Here's how the part is built. I have some questions about the finished solid (model axes, mm). A direction names the side the tool comes from. Round coordinates to 2 decimals unless told otherwise and drop trailing zeros. Write each loop counter-clockwise with the first axis right and the second up, starting at its lowest first coordinate (ties: lowest second). Pieces come first, ordered by that corner, then holes. Notation, with made-up numbers: M 33.5,38 L 62.5,38 A16 cw 62.5,64 Z; hole C -29.5,20 d1. An arc over 180 degrees is marked long. Use one line per item in the form item = value. Start each with the question number.
Q1. We'd pull the mould along X, two halves only. Please class faces 5 (the face through (-10, 82, -13)), 6 (the face through (60, 1, 0)), 7 (the face through (-1, 33, 22)): +X half, -X half, draft (parallel to the pull), parting line (faces both ways), or undercut.
Q2. For faces 1 (the face through (-42, 25, -5)), 2 (the face through (-45, 28, -6)), 3 (the face through (53, 3, 0)), 4 (the face through (-40, 66, -11)), which set-ups out of +Z, -Z, +X, -X, +Y, -Y let a thin tool reach every point of the face, with its end or its side?
Q3. I want a section at B-B on z = -17.5. List the corners of the cut face in (x, y) for me, and give its area (3 significant figures).
Q4. I want a section at C-C on y = 23. List the corners of the cut face in (x, z) for me.
Q5. I need wall thicknesses on line 1 along Z through (x, y) = (-52.5, 2.3); line 2 along X through (y, z) = (1.85, -17.5); line 3 along Y through (x, z) = (0, -24). Which ranges of each line are inside material? Lowest first, please. Write a range as from..to.
Q6. I'm going to push flat-ended pins straight in: pin 1 Ø8 at (y, z) = (14.5, -16) entering from +X; pin 2 Ø4 at (x, z) = (-42, 1.5) entering from +Y; pin 3 Ø10 at (y, z) = (37, -13.5) entering from -X. Where does each tip first touch, or does it pass through?
Q7. I want a section at D-D on z = 8. List the corners of the cut face in (x, y) for me (3 decimals), and give its area (3 significant figures).
Q8. I want a section at A-A on x = 52.5. List the corners of the cut face in (y, z) for me.
Autodesk Inventor part; units mm, degrees
ref_plane "YZ Plane" through (0, 0, 0) normal (1, 0, 0) x (0, 1, 0)
ref_plane "XZ Plane" through (0, 0, 0) normal (0, 1, 0) x (-1, 0, 0)
ref_plane "XY Plane" through (0, 0, 0) normal (0, 0, 1) x (1, 0, 0)
sketch "Skizze1" plane through (0, 0, 0) normal (0, 1, 0) x (-1, 0, 0)
  line L0 (60, 25) -> (-60, 25)
  line L1 (-60, 25) -> (-60, -25)
  line L2 (-60, -25) -> (60, -25)
  line L3 (60, -25) -> (60, 25)
  point P0 (0, 0)
  point P1 (0, 25)
  point P2 (-60, 0)
  dimension "d0" = 120
  dimension "d1" = 50
extrude "Extrusion1" add sketch "Skizze1" along normal blind 70
sketch "Skizze2" plane through (60, 0, 25) normal (1, 0, 0) x (0, 0, -1)
  line L0 (0, 0) -> (50, 0) construction
  line L1 (50, 0) -> (50, 70) construction
  line L2 (0, 70) -> (50, 70) construction
  line L3 (0, 0) -> (0, 70) construction
  line L4 (0, 70) -> (50, 70)
  line L5 (50, 70) -> (50, 3)
  line L6 (50, 3) -> (0, 3)
  line L7 (0, 3) -> (0, 70)
  line L8 (50, 0) -> (50, 70)
  point P0 (25, 0)
  dimension "d4" = 3
extrude "Extrusion2" cut sketch "Skizze2" against normal blind 15
sketch "Skizze3" plane through (-60, 0, -25) normal (-1, 0, 0) x (0, 0, 1)
  line L0 (0, 0) -> (50, 0) construction
  line L1 (50, 0) -> (50, 70) construction
  line L2 (0, 70) -> (50, 70) construction
  line L3 (0, 0) -> (0, 70) construction
  line L4 (0, 70) -> (50, 70)
  line L5 (50, 70) -> (50, 3)
  line L6 (50, 3) -> (0, 3)
  line L7 (0, 3) -> (0, 70)
  line L8 (50, 0) -> (50, 70)
  point P0 (25, 0)
  dimension "d7" = 3
extrude "Extrusion3" cut sketch "Skizze3" against normal blind 15
shell "Wandung1" thickness 3 removed faces 1 at (20, 0, 8.3333)
sketch "Skizze4" plane through (0, 0, 0) normal (0, -1, 0) x (1, 0, 0)
  line L0 (42, 22) -> (42, -22) construction
  line L1 (42, -22) -> (-42, -22) construction
  line L2 (-42, -22) -> (-42, 22) construction
  line L3 (-42, 22) -> (42, 22) construction
  line L4 (-60, 25) -> (60, 25) construction
  line L5 (-60, -25) -> (-60, 25) construction
  line L6 (60, -25) -> (-60, -25) construction
  line L7 (60, 25) -> (60, -25) construction
  line L8 (-84, 0) -> (84, 0) construction
  line L9 (0, -35) -> (0, 35) construction
  point P0 (0, 0)
  point P1 (-52.5, -17.5)
  point P2 (-52.5, 17.5)
  point P3 (52.5, 17.5)
  point P4 (52.5, -17.5)
  dimension "d11" = 7.5
  dimension "d12" = 7.5
hole "Bohrung1" at (-52.5, 0, -17.5) at (-52.5, 0, 17.5) at (52.5, 0, 17.5) at (52.5, 0, -17.5) direction (0, 1, 0) diameter 5.5 end through all
sketch "Skizze5" plane through (60, 0, -25) normal (0, 0, -1) x (-1, 0, 0)
  line L0 (120, 3) -> (105, 3)
  line L1 (105, 3) -> (105, 70)
  line L2 (15, 70) -> (105, 70)
  line L3 (15, 70) -> (15, 3)
  line L4 (15, 3) -> (0, 3)
  line L5 (0, 0) -> (0, 3)
  line L6 (0, 0) -> (120, 0)
  line L7 (120, 0) -> (120, 3)
  point P0 (60, 0)
  point P1 (60, 23)
  point P2 (60, 0)
  dimension "d20" = 23
hole "Bohrung2" at (0, 23, -25) direction (0, 0, 1) diameter 8.5 end through all
sketch "Skizze6" plane through (-60, 0, 25) normal (0, 0, 1) x (1, 0, 0)
  circle A0 centre (60, 23) radius 4.25 construction
  line L0 (15, 3) -> (0, 3) construction
  line L1 (0, 0) -> (0, 3) construction
  line L2 (0, 0) -> (120, 0) construction
  line L3 (120, 0) -> (120, 3) construction
  line L4 (120, 3) -> (105, 3) construction
  line L5 (105, 3) -> (105, 70) construction
  line L6 (15, 70) -> (105, 70) construction
  line L7 (15, 70) -> (15, 3) construction
  line L8 (15, 70) -> (60, 70)
  line L9 (60, 70) -> (15, 30)
  line L10 (15, 30) -> (15, 70)
  line L11 (15, 70) -> (15, 3)
  point P0 (60, 0)
  dimension "d28" = 45
  dimension "d29" = 30
extrude "Extrusion4" cut sketch "Skizze6" against normal blind 25
sketch "Skizze7" plane through (0, 70, 0) normal (0, 1, 0) x (1, 0, 0)
  line L0 (0, 0) -> (0, -25) construction
  line L1 (0, -25) -> (45, -25) construction
  line L2 (45, -25) -> (45, 25) construction
  line L3 (45, 25) -> (-45, 25) construction
  line L4 (-45, 25) -> (-45, 0) construction
  line L5 (-45, 0) -> (0, 0) construction
  circle A0 centre (-10, 12.5) radius 3
  circle A1 centre (30, 12.5) radius 3
  point P0 (0, 0)
  point P1 (-45, 12.5)
  dimension "d32" = 6
  dimension "d34" = 6
  dimension "d35" = 40
  dimension "d43" = 15
extrude "Extrusion5" add sketch "Skizze7" along normal blind 12
thread "Gewinde1"
thread "Gewinde2"
fillet "Rundung1" radius 5 4 edges at (42, 67, 0) (-42, 67, -11) (-45, 70, -12.5) (45, 70, 0)
properties part number "Radkasten_Links"
Reported:
q1.face_5 = draft
q1.face_6 = +X half
q1.face_7 = undercut
q2.face_1 = -Y
q2.face_2 = +Z, -Z, -X, +Y
q2.face_3 = +Z, -Z, +X, +Y
q2.face_4 = +Z, -Y
q3.outline = M -60,0 L -55.25,0 L -55.25,3 L -60,3 Z; M -49.75,0 L -42,0 L -42,62 A5 cw -37,67 L 37,67 A5 cw 42,62 L 42,0 L 49.75,0 L 49.75,3 L 45,3 L 45,65 A5 ccw 40,70 L -40,70 A5 ccw -45,65 L -45,3 L -49.75,3 Z; M 55.25,0 L 60,0 L 60,3 L 55.25,3 Z
q3.area = 729 mm^2
q4.outline = M -45,-25 L -4.25,-25 L -4.25,-22 L -42,-22 L -42,22 L -4.25,22 L -4.25,25 L -45,25 Z; M 4.25,-25 L 45,-25 L 45,25 L 4.25,25 L 4.25,22 L 42,22 L 42,-22 L 4.25,-22 Z
q5.line_1 = -25..-20.25, -14.75..14.75, 20.25..25
q5.line_2 = -60..-55.25, -49.75..-42, 42..49.75, 55.25..60
q5.line_3 = 0..18.75, 27.25..70
q6.pin_1 = 45
q6.pin_2 = 69.95
q6.pin_3 = -45
q7.outline = M -60,0 L -42,0 L -42,32.667 L -45,30 L -45,3 L -60,3 Z; M -3.375,67 L 37,67 A5 cw 42,62 L 42,0 L 60,0 L 60,3 L 45,3 L 45,65 A5 ccw 40,70 L 0,70 Z
q7.area = 525 mm^2
q8.outline = M 0,-25 L 3,-25 L 3,-20.25 L 0,-20.25 Z; M 0,-14.75 L 3,-14.75 L 3,14.75 L 0,14.75 Z; M 0,20.25 L 3,20.25 L 3,25 L 0,25 Z
